Input: part model. Units: mm. Frame: model coordinates. Face numbers are marked on the shaded views. A direction names the side the tool comes from. Coordinates: 2 decimals unless noted, no trailing zeros. Loops run counter-clockwise (first coordinate to the right, second up) from the corner with the lowest first, then second, coordinate; pieces in that order, holes last. Notation, with made-up numbers: (-14, 67) - (4, 67) arc R23 ccw to (4, 89) - close; hole circle Ø6 at (63, 26). An arc over 180 degrees is marked (long way). Use one line per item in the form item = value.
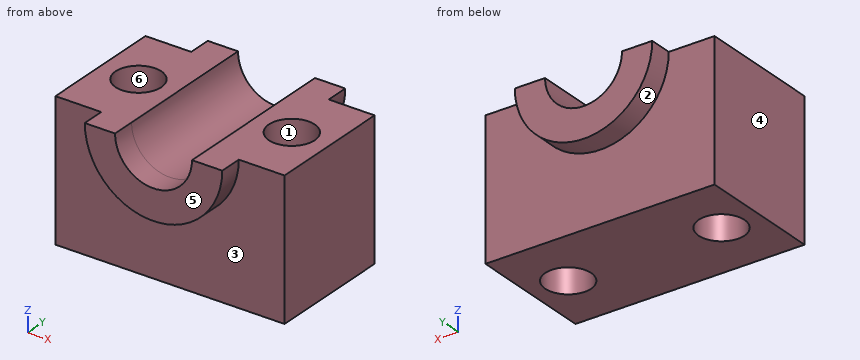
from build123d import *

# Parameters (mm, degrees)
F1_DEPTH = 76.2
F3_DEPTH = 12.7
F4_R     = 21.3338739626
F5_DEPTH = 101.6
F7_DEPTH = 12.7
F9_DEPTH = 127


with BuildPart() as f1:
    # F0 (on Top) → F1 (new body)
    with BuildSketch(Plane.XY):
        Polygon((38.1, -34.6363636543), (63.5, -34.6363636543), (63.5, 34.6363636543), (38.1, 34.6363636543), (38.1, 47.3363636543), (-38.1, 47.3363636543), (-38.1, 34.6363636543), (-63.5, 34.6363636543), (-63.5, -34.6363636543), (-38.1, -34.6363636543), (-38.1, -47.3363636543), (38.1, -47.3363636543), align=None)
    extrude(amount=F1_DEPTH)

    # F2 (on face) → F3 (cut)
    with BuildSketch(Plane.XZ.offset(47.3363636543)):
        with BuildLine():
            Line((38.1, 0), (38.1, 76.2))
            ThreePointArc((38.1, 76.2), (0, 38.1), (-38.1, 76.2))
            Line((-38.1, 76.2), (-38.1, 0))
            Line((-38.1, 0), (38.1, 0))
        make_face()
        with BuildLine():
            Line((21.3338739626, 76.2), (38.1, 76.2))
            ThreePointArc((38.1, 76.2), (0, 114.3), (-38.1, 76.2))
            Line((-38.1, 76.2), (-21.3338739626, 76.2))
            ThreePointArc((-21.3338739626, 76.2), (0, 97.5338739626), (21.3338739626, 76.2))
        make_face()
        with BuildLine():
            ThreePointArc((-21.3338739626, 76.2), (0, 54.8661260374), (21.3338739626, 76.2))
            Line((21.3338739626, 76.2), (-21.3338739626, 76.2))
        make_face()
    extrude(amount=-F3_DEPTH, mode=Mode.SUBTRACT)

    # F4 (on face) → F5 (cut)
    with BuildSketch(Plane.XZ.offset(34.6363636543)):
        with Locations((0, 76.2)):
            Circle(F4_R)
    extrude(amount=-F5_DEPTH, mode=Mode.SUBTRACT)

    # F6 (on face) → F7 (cut)
    with BuildSketch(Plane(origin=(0, 47.3363636543, 0), x_dir=(-1, 0, 0), z_dir=(0, 1, 0))):
        with BuildLine():
            ThreePointArc((38.1, 76.2), (0, 38.1), (-38.1, 76.2))
            Line((-38.1, 76.2), (-38.1, 0))
            Line((-38.1, 0), (38.1, 0))
            Line((38.1, 0), (38.1, 76.2))
        make_face()
    extrude(amount=-F7_DEPTH, mode=Mode.SUBTRACT)

    # F8 (on face) → F9 (cut)
    with BuildSketch(Plane.XY.offset(76.2)):
        with BuildLine():
            Line((55.2647357479, 0), (29.8647357479, 0))
            ThreePointArc((29.8647357479, 0), (42.5647357479, -12.7), (55.2647357479, 0))
        make_face()
        with BuildLine():
            ThreePointArc((55.2647357479, 0), (42.5647357479, 12.7), (29.8647357479, 0))
            Line((29.8647357479, 0), (55.2647357479, 0))
        make_face()
        with BuildLine():
            ThreePointArc((-55.1169369813, 0), (-42.4169369813, -12.7), (-29.7169369813, 0))
            Line((-29.7169369813, 0), (-55.1169369813, 0))
        make_face()
        with BuildLine():
            Line((-55.1169369813, 0), (-29.7169369813, 0))
            ThreePointArc((-29.7169369813, 0), (-42.4169369813, 12.7), (-55.1169369813, 0))
        make_face()
    extrude(amount=-F9_DEPTH, mode=Mode.SUBTRACT)


solid = f1.part
Q1. Cut plane A-A, the plane y = 0. Return loops of the section in (x, z).
Check values:
outline = (-63.5, 0) - (-55.12, 0) - (-55.12, 76.2) - (-63.5, 76.2) - close; (-29.72, 0) - (29.86, 0) - (29.86, 76.2) - (21.33, 76.2) arc R21.33 cw to (-21.33, 76.2) - (-29.72, 76.2) - close; (55.26, 0) - (63.5, 0) - (63.5, 76.2) - (55.26, 76.2) - close
Q2. Ray query, line 1 along Y through (x, z) = (-47, 65.5); line 2 along Y through (x, z) = (18, 13); line 3 along Y through (x, z) = (-46.5, 3). Return the intervals inside material, ascending. Write a range as [from, to].
Check values:
line_1 = [-34.64, -11.84], [11.84, 34.64]
line_2 = [-34.64, 34.64]
line_3 = [-34.64, -12.03], [12.03, 34.64]
Q3. First-contact query: P1, Ø3, axis at x = 39.5, z = 17.5, coming from the -Y side; P2, Ø6, axis at y = 36, z = 15, coming from the -X side; P3, Ø15, axis at x = -42.42, y = 0, coming from the +Z side; P4, Ø8, axis at x = -44, z = 56, coming from the +Y side. Flat tips, straight axial feed; report the tip coordinate or a pass-through.
Check values:
P1 = -34.64
P2 = -63.5
P3 = through
P4 = 34.64
Q4. Pull-direction query (X, two-part tool) for the marked faces 4, 5 and 6; classes: pulls with the +X half, pulls with the -X half, needs draft (parallel to the pull), parting line crosses it, or undercut.
Check values:
face_4 = pulls with the -X half
face_5 = needs draft
face_6 = undercut
Q5. Cut plane B-B, the plane z = 63.5. Return loops of the section in (x, y).
Check values:
outline = (-63.5, -34.64) - (-35.92, -34.64) - (-35.92, -47.34) - (-17.14, -47.34) - (-17.14, 47.34) - (-35.92, 47.34) - (-35.92, 34.64) - (-63.5, 34.64) - close; (17.14, -47.34) - (35.92, -47.34) - (35.92, -34.64) - (63.5, -34.64) - (63.5, 34.64) - (35.92, 34.64) - (35.92, 47.34) - (17.14, 47.34) - close; hole circle Ø25.4 at (-42.42, 0); hole circle Ø25.4 at (42.56, 0)
Q6. Set-up query: the marked faces 1, 2 and 3. Return all of +Z, -Z, +X, -X, +Y, -Y with unobstructed straight access to the full face (end or side cutting, diameter ignored); none if empty.
Check values:
face_1 = +Z, -Z
face_2 = -Z, +Y
face_3 = -Z, -Y
Q7. Cut plane D-D, the plane z = 35. Return loops of the section in (x, y).
Check values:
outline = (-63.5, -34.64) - (63.5, -34.64) - (63.5, 34.64) - (-63.5, 34.64) - close; hole circle Ø25.4 at (-42.42, 0); hole circle Ø25.4 at (42.56, 0)
Q8. Cut plane C-C, the plane x = 0. Return loops of the section in (y, z), then the cut area to 3 significant figures.
Check values:
outline = (-47.34, 38.1) - (-34.64, 38.1) - (-34.64, 0) - (34.64, 0) - (34.64, 38.1) - (47.34, 38.1) - (47.34, 54.87) - (-47.34, 54.87) - close
area = 4,230 mm²
